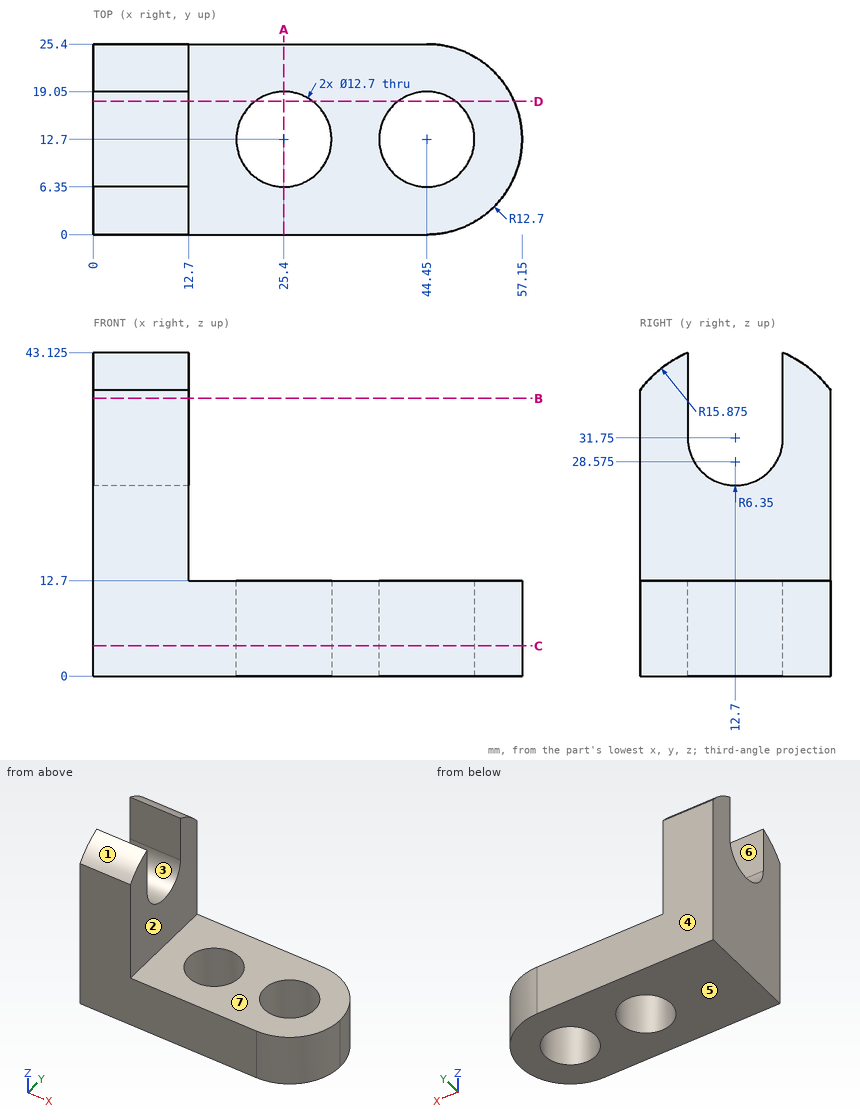
Design review of the part shown in the three views and the two pictorial views. Dimensions are in mm from the part's minimum x, y and z. A direction names the side the tool comes from. Round coordinates to 2 decimals unless told otherwise and drop trailing zeros. Order: outer loops, then holes, each group sorted by start corner. A loop starts at its lowest first (then second) coordinate and runs counter-clockwise, first axis right, second up.
Q1. We need section B-B, the plane z = 37. Give the boundary of the cut face in (x, y).
Findings below:
outline: (0, 0) - (12.7, 0) - (12.7, 6.35) - (0, 6.35) - close; (0, 19.05) - (12.7, 19.05) - (12.7, 25.4) - (0, 25.4) - close
Q2. Insertion check: P1, Ø7.5, axis at x = 29, y = 9.5, coming from the +Z side; P2, Ø12.5, axis at y = 18, z = 28.5, coming from the +X side. Each pin has a flat end and moves straight along its axis. Give the tip position at first contact, or say it passes through.
Findings below:
P1: stops at z = 12.7
P2: stops at x = 12.7
Q3. Wall thickness on line 1 (Y direction, x = 6, z = 36); line 2 (X direction, y = 11, z = 8) (1 decimal): over which ranges is each line inside the solid? List them lowest first.
Findings below:
line 1: y = 0 to 6.35, 19.05 to 25.4
line 2: x = 0 to 19.3, 31.5 to 38.3, 50.6 to 57
Q4. Mouldability with a two-part tool opening along Y and no side actions: class the marked faces 1, 2, 3 and 4 as pulls with the +Y half, pulls with the -Y half, needs draft (parallel to the pull), parting line crosses it, or undercut.
Findings below:
face 1: pulls with the -Y half
face 2: needs draft
face 3: undercut
face 4: pulls with the +Y half
Q5. We need section A-A, the plane x = 25.4. Give the boundary of the cut face in (y, z), plus the area to 3 significant figures.
Findings below:
outline: (0, 0) - (6.35, 0) - (6.35, 12.7) - (0, 12.7) - close; (19.05, 0) - (25.4, 0) - (25.4, 12.7) - (19.05, 12.7) - close
area: 161 mm2
Q6. We need section D-D, the plane y = 17.75. Give the boundary of the cut face in (x, z), plus the area to 3 significant figures.
Findings below:
outline: (0, 0) - (21.55, 0) - (21.55, 12.7) - (12.7, 12.7) - (12.7, 27.9) - (0, 27.9) - close; (29.25, 0) - (40.6, 0) - (40.6, 12.7) - (29.25, 12.7) - close; (48.3, 0) - (56.1, 0) - (56.1, 12.7) - (48.3, 12.7) - close
area: 710 mm2
Q7. Machinability: for the marked faces 5, 6 and 7, which of the approach directions +Z, -Z, +X, -X, +Y, -Y give a long, thin tool a straight path to every point of the face, cutting with its end or side? Answer none if there is none.
Findings below:
face 5: -Z, +X, -X, +Y, -Y
face 6: +Z, +X, -X
face 7: +Z, +X, +Y, -Y
Q8. We need section C-C, the plane z = 4. Give the boundary of the cut face in (x, y), plus the area to 3 significant figures.
Findings below:
outline: (0, 0) - (44.45, 0) arc R12.7 ccw to (44.45, 25.4) - (0, 25.4) - close; hole circle Ø12.7 at (25.4, 12.7); hole circle Ø12.7 at (44.45, 12.7)
area: 1,130 mm2
